Could you check a few things on this model? Use its own coordinates, in mm. Face numbers are marked on the shaded views. Give positions to 0.01 mm unless a question says otherwise; leave off trailing zeros. Loops run counter-clockwise (first coordinate to the right, second up) from the corner with the lowest first, then second, coordinate; pieces in that order, holes last. Notation, with made-up numbers: M 82,-4 L 136,-4 A27 cw 136,18 Z; hole C -33.75,82 d2. An arc over 180 degrees is marked long. Answer in a Markdown table with one row per item. Add a question column.
1. I need wall thicknesses on line 1 along X through (y, z) = (6, 26); line 2 along Y through (x, z) = (5, -3.5); line 3 along Y through (x, z) = (1, 23.5). Which ranges of each line are inside material? Lowest first, please. Write a range as from..to.
2. If we section it at C-C on y = 6: Count the separate pieces of the cut face and the enclosed holes in it, then the cut area to 3 significant figures.
3. If we section it at D-D on z = 25.5: List the corners of the cut face in (x, y) for me.
4. I'm going to push flat-ended pins straight in: pin 1 Ø6 at (x, z) = (1.5, 48) entering from -Y; pin 2 Ø3 at (x, z) = (-7.5, 19.5) entering from +Y; pin 3 Ø0.9 at (x, y) = (2, 28) entering from +Z; pin 4 Ø1.5 at (y, z) = (6.5, 21) entering from +X. Where does each tip first touch, or does it pass through?
5. Thinking about a two-plate mould opening in X: for the marked faces 1 and 2, which applies, released by +X, released by -X, zero draft, split by the parting line, or undercut?
6. If we section it at A-A on y = 9.5: List the corners of the cut face in (x, z) for me.
7. If we section it at B-B on x = -1: List the corners of the cut face in (y, z) for me.
```python
from build123d import *

# Parameters (mm, degrees)
SKETCH1_W                   = 32
SKETCH1_H                   = 75
BOSS_EXTRUDE1_DEPTH         = 5
SKETCH5_W                   = 2.5
SKETCH5_H                   = 5
BOSS_EXTRUDE2_DEPTH         = 26
SKETCH7_W                   = 5
SKETCH7_H                   = 5
BOSS_EXTRUDE3_DEPTH         = 27
SKETCH8_W                   = 11
SKETCH8_H                   = 5
CUT_EXTRUDE1_DEPTH          = 1.5
SKETCH9_W                   = 3
SKETCH9_H                   = 3
BOSS_EXTRUDE4_DEPTH         = 4
SKETCH10_R                  = 1.25
CUT_EXTRUDE2_DEPTH          = 3
SKETCH11_W                  = 5.5
SKETCH11_H                  = 75
BOSS_EXTRUDE5_DEPTH         = 2
TAP_DRILL_FOR_M3X0_5_TAP1_D = 2.5


with BuildPart() as part:
    # Sketch1 → Boss-Extrude1 (new body)
    with BuildSketch(Plane(origin=(0, 0, 0), x_dir=(1, 0, 0), z_dir=(0, 1, 0))):
        with Locations((2.576120431, -29.854896849)):
            Rectangle(SKETCH1_W, SKETCH1_H)
    extrude(amount=BOSS_EXTRUDE1_DEPTH)

    # Sketch5 → Boss-Extrude2 (add)
    with BuildSketch(Plane(origin=(0, 5, 0), x_dir=(1, 0, 0), z_dir=(0, 1, 0))):
        with Locations((-12.173879569, 5.145103151)):
            Rectangle(SKETCH5_W, SKETCH5_H)
        with Locations((17.326120431, 5.145103151)):
            Rectangle(SKETCH5_W, SKETCH5_H)
    extrude(amount=BOSS_EXTRUDE2_DEPTH)

    # Sketch7 → Boss-Extrude3 (add)
    with BuildSketch(Plane.ZY.offset(-16.076120431)):
        with Locations((-5.145103151, 28.5)):
            Rectangle(SKETCH7_W, SKETCH7_H)
    extrude(amount=BOSS_EXTRUDE3_DEPTH)

    # Sketch8 → Cut-Extrude1 (cut)
    with BuildSketch(Plane(origin=(0, 0, -7.645103151), x_dir=(-1, 0, 0), z_dir=(0, 0, -1))):
        with Locations((-2.576120431, 28.5)):
            Rectangle(SKETCH8_W, SKETCH8_H)
    extrude(amount=-CUT_EXTRUDE1_DEPTH, mode=Mode.SUBTRACT)

    # Sketch9 → Boss-Extrude4 (add)
    with BuildSketch(Plane.XY.offset(-2.645103151)):
        with Locations((2.576120431, 27.5)):
            Rectangle(SKETCH9_W, SKETCH9_H)
    extrude(amount=BOSS_EXTRUDE4_DEPTH)

    # Sketch10 → Cut-Extrude2 (cut)
    with BuildSketch(Plane(origin=(0, 26, 0), x_dir=(-1, 0, 0), z_dir=(0, -1, 0))):
        with Locations((-2.576120431, 0.645103151)):
            Circle(SKETCH10_R)
    extrude(amount=-CUT_EXTRUDE2_DEPTH, mode=Mode.SUBTRACT)

    # Sketch11 → Boss-Extrude5 (add)
    with BuildSketch(Plane(origin=(0, 5, 0), x_dir=(1, 0, 0), z_dir=(0, 1, 0))):
        with Locations((-6.673879569, -29.854896849)):
            Rectangle(SKETCH11_W, SKETCH11_H)
        with Locations((11.826120431, -29.854896849)):
            Rectangle(SKETCH11_W, SKETCH11_H)
    extrude(amount=BOSS_EXTRUDE5_DEPTH)

    # Tap Drill for M3x0.5 Tap1 (through all)
    with Locations(Plane(origin=(12.076120431, 0, 59.854896849), x_dir=(0, 0, -1), z_dir=(0, -1, 0))):
        with Locations((0, 0), (15, 0), (30, 0), (45, 0), (60, 0), (0, -19), (15, -19), (30, -19), (45, -19), (60, -19)):
            Hole(TAP_DRILL_FOR_M3X0_5_TAP1_D / 2)


solid = part.part
```
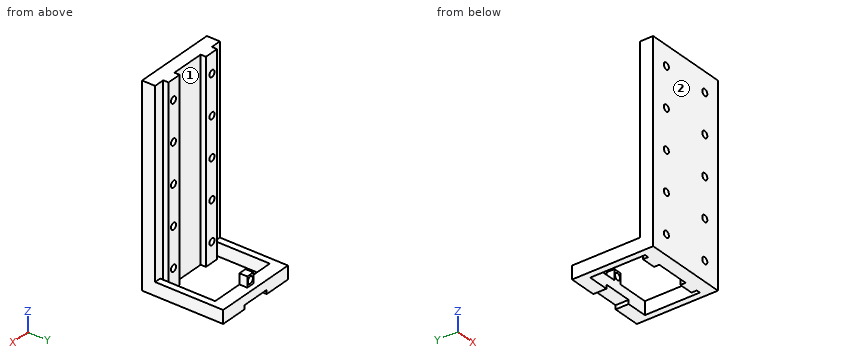
Results:
| question | item | result |
|---|---|---|
| 1 | line 1 | -9.42..-3.92, 9.08..14.58 |
| 1 | line 2 | 0..5, 26..31 |
| 1 | line 3 | 0..5 |
| 2 | separate pieces | 4 |
| 2 | enclosed holes | 10 |
| 2 | area | 801 mm2 |
| 3 | outline | M -13.42,0 L 18.58,0 L 18.58,5 L 14.58,5 L 14.58,7 L 9.08,7 L 9.08,5 L -3.92,5 L -3.92,7 L -9.42,7 L -9.42,5 L -13.42,5 Z |
| 4 | pin 1 | y = 0 |
| 4 | pin 2 | y = 7 |
| 4 | pin 3 | z = 1.35 |
| 4 | pin 4 | x = 14.58 |
| 5 | face 1 | undercut |
| 5 | face 2 | zero draft |
| 6 | outline | M -13.42,-7.65 L -10.92,-7.65 L -10.92,-2.65 L -13.42,-2.65 Z; M 16.08,-7.65 L 18.58,-7.65 L 18.58,-2.65 L 16.08,-2.65 Z |
| 7 | outline | M 0,-7.65 L 5,-7.65 L 5,67.35 L 0,67.35 Z; M 26,-6.15 L 31,-6.15 L 31,-2.65 L 26,-2.65 Z |
